Source: CAD feature listing. Evaluate the final solid. Frame: model axes, mm. Coordinates: 2 decimals unless noted, no trailing zeros. Write each loop counter-clockwise with the first axis right and the second up, starting at its lowest first coordinate (ties: lowest second). Pieces come first, ordered by that corner, then holes. Notation, with made-up numbers: (83.25, 77) -> (94.25, 77) arc R31 cw to (94.25, 109) -> close; hole circle Ø7 at (28.5, 70.25). An arc over 180 degrees is marked (long way). One line per item, written item: value. Start each with the question number.
1. Section query A-A, the plane z = 37.5. Output: boundary loops of the cut face in (x, y), and give its area (3 significant figures).
2. Line query: line 1 (Y direction, x = 0, z = 15.6); line 2 (Y direction, x = 0, z = 7); line 3 (Z direction, x = 1.75, y = 1.75). Output: solid intervals per line, ascending.
3. First-contact query: P1, Ø3, axis at x = 4, z = 30, coming from the -Y side; P2, Ø1.5, axis at x = -3, z = 12, coming from the +Y side; P3, Ø1.5, axis at x = 0.5, y = 0, coming from the -Z side. Flat tips, straight axial feed; report the tip coordinate or a pass-through.
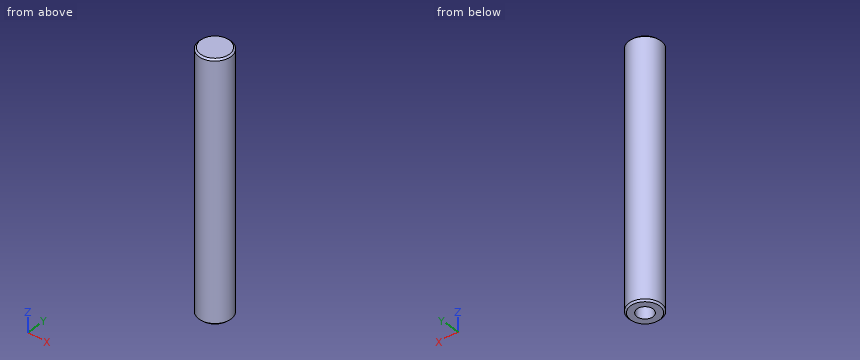
from build123d import *

# Parameters (mm, degrees)
SKETCH_1_R                   = 5
EXTRUDE_1_DEPTH              = 80
HOLE_WIZARD_M5_1_D           = 4.2
HOLE_WIZARD_M5_1_DEPTH       = 17.4
HOLE_WIZARD_M5_1_CBORE_D     = 5
HOLE_WIZARD_M5_1_CBORE_DEPTH = 15
HOLE_WIZARD_M5_1_TIP         = 1.2618073
CHAMFER_1_SIZE               = 0.5


with BuildPart() as part:
    # 草图1 → 拉伸1 (new body)
    with BuildSketch(Plane.XY):
        Circle(SKETCH_1_R)
    extrude(amount=EXTRUDE_1_DEPTH)

    # M5 螺纹孔1
    with Locations(Plane(origin=(0, 0, 0), x_dir=(-1, 0, 0), z_dir=(0, 0, -1))):
        with Locations((0, 0)):
            CounterBoreHole(HOLE_WIZARD_M5_1_D / 2, HOLE_WIZARD_M5_1_CBORE_D / 2, HOLE_WIZARD_M5_1_CBORE_DEPTH, depth=HOLE_WIZARD_M5_1_DEPTH)
            with Locations((0, 0, -(HOLE_WIZARD_M5_1_DEPTH + HOLE_WIZARD_M5_1_TIP / 2))):  # 118° drill point
                Cone(0, HOLE_WIZARD_M5_1_D / 2, HOLE_WIZARD_M5_1_TIP, mode=Mode.SUBTRACT)

    # 倒角1
    chamfer_1_edges = [part.edges().sort_by_distance(p)[0] for p in [
        (-5, 0, 0),
        (-5, 0, 80),
    ]]
    chamfer(chamfer_1_edges, length=CHAMFER_1_SIZE)


solid = part.part
Computed values:
1. outline: circle Ø10 at (0, 0)
1. area: 78.5 mm²
2. line 1: y = -5 to -2.1, 2.1 to 5
2. line 2: y = -5 to -2.5, 2.5 to 5
2. line 3: z = 15 to 80
3. P1: stops at y = -4.33
3. P2: stops at y = 4.47
3. P3: stops at z = 17.91
